Source: three-view drawing plus pictorial views. Frame: mm from the lowest corner of the part. Give positions to 0.01 mm unless a question says otherwise; leave off trailing zeros. Loops run counter-clockwise (first coordinate to the right, second up) from the corner with the lowest first, then second, coordinate; pieces in that order, holes last. Notation, with made-up numbers: (0.25, 42.5) -> (54.25, 42.5) arc R26 ccw to (54.25, 74.5) -> close; hole circle Ø11 at (26.25, 37). An arc over 180 degrees is marked (long way). Answer in a Markdown table with one row per item. Add a question column.
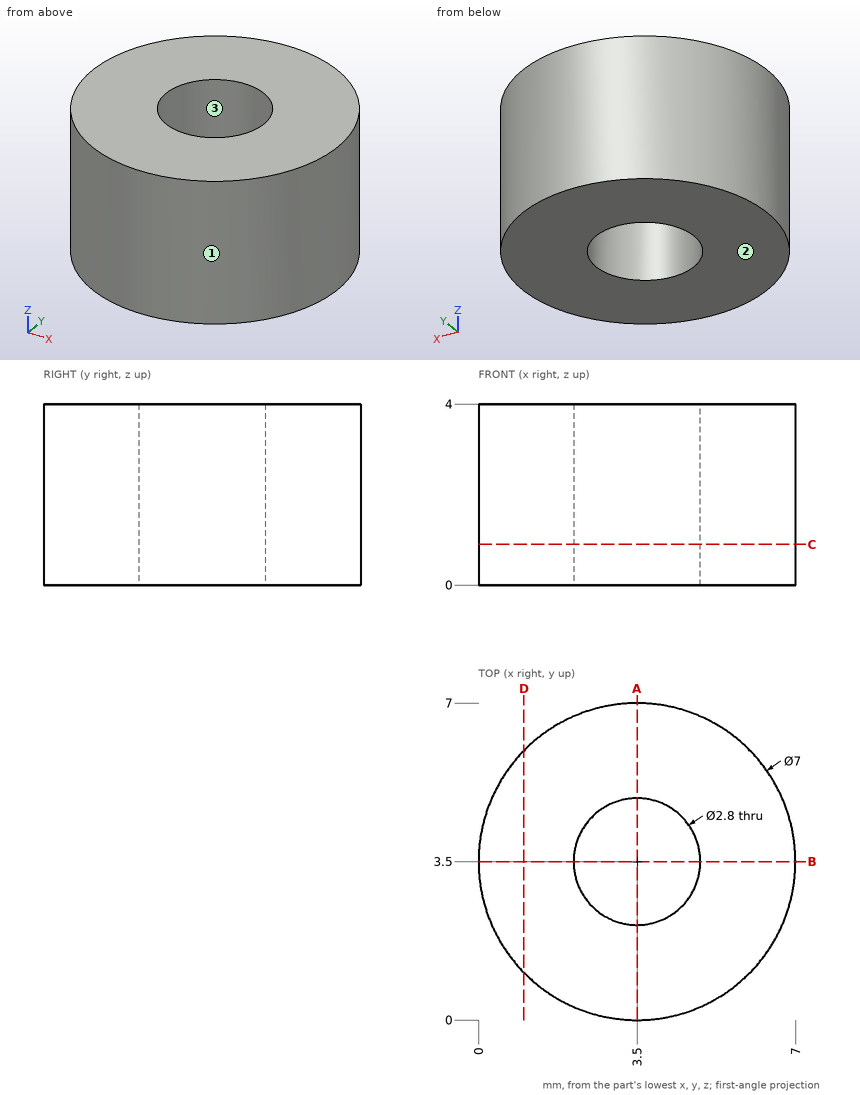
(1) Cut plane A-A on x = 3.5. Return the cut outline in (y, z), then the cut area to 3 significant figures.
(2) Draft query along X for the marked faces 1, 2 and 3. Return one class per face: +X half, -X half, draft (parallel to the pull), parting line (faces both ways), or undercut.
(3) Cut plane C-C on z = 0.9. Return the cut outline in (x, y).
(4) Material intervals for line 1 along Y through (x, z) = (3.5, 2.8); line 2 along X through (y, z) = (3.25, 2.85); line 3 along Y through (x, z) = (4.5, 0.45), sorted ascending. Write a range as from..to.
(5) Cut plane D-D on x = 1. Return the cut outline in (y, z).
Answer list:
| question | item | result |
|---|---|---|
| 1 | outline | (0, 0) -> (2.1, 0) -> (2.1, 4) -> (0, 4) -> close; (4.9, 0) -> (7, 0) -> (7, 4) -> (4.9, 4) -> close |
| 1 | area | 16.8 mm² |
| 2 | face 1 | parting line |
| 2 | face 2 | draft |
| 2 | face 3 | undercut |
| 3 | outline | circle Ø7 at (3.5, 3.5); hole circle Ø2.8 at (3.5, 3.5) |
| 4 | line 1 | y = 0..2.1, 4.9..7 |
| 4 | line 2 | x = 0.01..2.12, 4.88..6.99 |
| 4 | line 3 | y = 0.15..2.52, 4.48..6.85 |
| 5 | outline | (1.05, 0) -> (5.95, 0) -> (5.95, 4) -> (1.05, 4) -> close |
